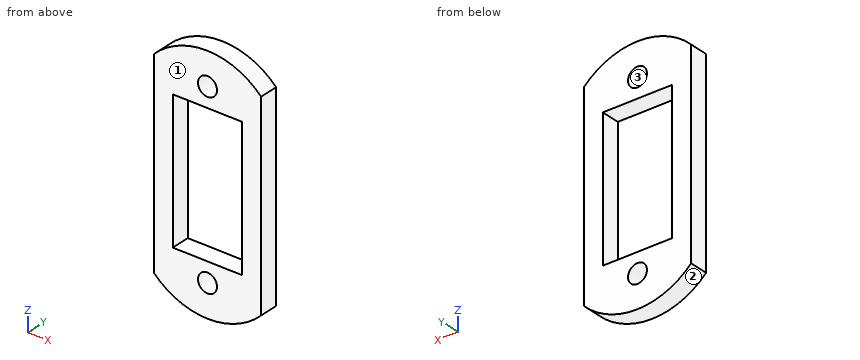
Autodesk Inventor part; units mm, degrees
ref_plane "YZ Plane" through (0, 0, 0) normal (1, 0, 0) x (0, 1, 0)
ref_plane "XZ Plane" through (0, 0, 0) normal (0, 1, 0) x (-1, 0, 0)
ref_plane "XY Plane" through (0, 0, 0) normal (0, 0, 1) x (1, 0, 0)
sketch "Sketch1" plane through (0, 0, 0) normal (0, 1, 0) x (-1, 0, 0)
  line L0 (9.2564, 10.8677) -> (9.2564, -11.1323)
  line L1 (9.2564, -11.1323) -> (-1.7436, -11.1323)
  line L2 (-1.7436, -11.1323) -> (-1.7436, 10.8677)
  line L3 (-1.7436, 10.8677) -> (9.2564, 10.8677)
  line L4 (12.2564, -15.8323) -> (12.2564, 15.5677)
  line L5 (-4.7436, 15.5677) -> (-4.7436, -15.8323)
  arc A0 (12.2564, 15.5677) -> (-4.7436, 15.5677) centre (3.7564, 7.0972) ccw
  arc A1 (-4.7436, -15.8323) -> (12.2564, -15.8323) centre (3.7564, -7.3617) ccw
  circle A2 centre (3.7564, 13.9677) radius 1.5
  circle A3 centre (3.7564, -14.2323) radius 1.5
  point P0 (0, 0)
  dimension "d0" = 22
extrude "Extrusion1" add sketch "Sketch1" along normal blind 3
properties part number "servo Holder" material "ABS Plastic"
Source: CAD feature listing. Evaluate the final solid. Frame: model axes, mm. Face numbers are marked on the shaded views. Round coordinates to 2 decimals unless told otherwise and drop trailing zeros. Loops run counter-clockwise (first coordinate to the right, second up) from the corner with the lowest first, then second, coordinate; pieces in that order, holes last. Notation, with made-up numbers: (79.25, 34) - (126.25, 34) arc R13 cw to (126.25, 48) - close; hole circle Ø8 at (63, 86). An arc over 180 degrees is marked (long way). Write item = value, one per line. Start each with the question number.
Item 1: Section query A-A on x = 1.25. Output: boundary loops of the cut face in (y, z).
Item 2: Section query D-D on x = -3. Output: boundary loops of the cut face in (y, z), plus the area to 3 significant figures.
Item 3: Section query B-B on z = 6. Output: boundary loops of the cut face in (x, y).
Item 4: Section query C-C on y = 2.25. Output: boundary loops of the cut face in (x, z), plus the area to 3 significant figures.
Item 5: Mould query, pull axis X, two halves, no side actions, for the marked faces 1, 2 and 3. Classes: released by +X, released by -X, zero draft, split by the parting line, or undercut.
Item 6: Material intervals for line 1 (X direction, y = 2.5, z = -6); line 2 (Z direction, x = -4.5, y = 1.6); line 3 (Z direction, x = -3.5, y = 0.3), sorted ascending.
Item 7: First-contact query: pin 1 Ø1.5 at (x, y) = (-1, 1) entering from -Z; pin 2 Ø1.5 at (x, y) = (0.5, 1) entering from -Z. Flat tips, straight axial feed; report the tip coordinate or a pass-through.
Results list:
q1.outline = (0, -18.27) - (3, -18.27) - (3, -11.13) - (0, -11.13) - close; (0, 10.87) - (3, 10.87) - (3, 18) - (0, 18) - close
q2.outline = (0, -19.34) - (3, -19.34) - (3, -15.53) - (0, -15.53) - close; (0, -12.94) - (3, -12.94) - (3, -11.13) - (0, -11.13) - close; (0, 10.87) - (3, 10.87) - (3, 12.67) - (0, 12.67) - close; (0, 15.26) - (3, 15.26) - (3, 19.07) - (0, 19.07) - close
q2.area = 33.7 mm²
q3.outline = (-12.26, 0) - (-9.26, 0) - (-9.26, 3) - (-12.26, 3) - close; (1.74, 0) - (4.74, 0) - (4.74, 3) - (1.74, 3) - close
q4.outline = (-12.26, -15.83) arc R12 ccw to (4.74, -15.83) - (4.74, 15.57) arc R12 ccw to (-12.26, 15.57) - close; hole (-9.26, -11.13) - (1.74, -11.13) - (1.74, 10.87) - (-9.26, 10.87) - close; hole circle Ø3 at (-3.76, -14.23); hole circle Ø3 at (-3.76, 13.97)
q4.area = 360 mm²
q5.face_1 = zero draft
q5.face_2 = split by the parting line
q5.face_3 = undercut
q6.line_1 = -12.26 to -9.26, 1.74 to 4.74
q6.line_2 = -19.34 to -15.54, -12.93 to -11.13, 10.87 to 12.66, 15.27 to 19.07
q6.line_3 = -19.36 to -15.71, -12.75 to -11.13, 10.87 to 12.49, 15.45 to 19.09
q7.pin_1 = -19.19
q7.pin_2 = -18.84
